Design review of the part built by this model. Coordinates are the model's own, in mm. A direction names the side the tool comes from. Give positions to 0.01 mm unless a question says otherwise; leave off trailing zeros. Write each loop counter-clockwise with the first axis right and the second up, starting at its lowest first coordinate (ties: lowest second). Pieces come first, ordered by that corner, then holes.
```python
from build123d import *

# Parameters (mm, degrees)
FILETE1_R = 2


with BuildPart() as part:
    # Esboço1 → Revolução1 (revolve)
    with BuildSketch(Plane.XY):
        Polygon((0, 31.5), (8, 31.5), (8, 27.5), (6, 27.5), (6, 0), (4, 0), (4, -21.5), (3.090074414, -24), (0, -24), align=None)
    revolve(axis=Axis((0, -53.197951274, 0), (0, 1, 0)))

    # Filete1
    filete1_edges = [part.edges().sort_by_distance(p)[0] for p in [
        (-8, 31.5, 0),
    ]]
    fillet(filete1_edges, radius=FILETE1_R)


solid = part.part
```
(1) Clearance check with flat-ended pins moving along their axes: P1, Ø4, axis at x = -6, y = 17.5, coming from the +Z side; P2, Ø5, axis at y = 16, z = -6, coming from the +X side; P3, Ø5, axis at y = 2, z = -2, coming from the +X side. State where each tip first meets the part, or that it passes through.
Resolved:
P1: stops at z = 4.47
P2: stops at x = 4.87
P3: stops at x = 6
(2) Consider section D-D, the plane y = 20. Give the boundary of the cut face in (x, z), then the cut area to 3 significant figures.
Resolved:
outline: circle Ø12 at (0, 0)
area: 113 mm2
(3) To check wall thickness, follow L1, parallel to Y at x = -0.5, z = -4.5; L2, parallel to X at y = -16.5, z = -2.75; L3, parallel to Z at x = -2.5, y = 12.5. State the ranges of each line that lie inside material, in increasing order.
Resolved:
L1: y = 0 to 31.5
L2: x = -2.9 to 2.9
L3: z = -5.45 to 5.45
(4) Consider section A-A, the plane z = 0. Give the boundary of the cut face in (x, y).
Resolved:
outline: (-8, 27.5) - (-6, 27.5) - (-6, 0) - (-4, 0) - (-4, -21.5) - (-3.09, -24) - (3.09, -24) - (4, -21.5) - (4, 0) - (6, 0) - (6, 27.5) - (8, 27.5) - (8, 29.5) arc R2 ccw to (6, 31.5) - (-6, 31.5) arc R2 ccw to (-8, 29.5) - close
(5) Tool access review of faces 1 (the face through (-6, 14, 0)), 2 (the face through (0, 31.5, 0)): name each direction out of +Z, -Z, +X, -X, +Y, -Y from which nothing blocks a thin tool from reaching the whole face with its end or side.
Resolved:
face 1: -Y
face 2: +Z, -Z, +X, -X, +Y
(6) Consider section C-C, the plane y = -15. Give the boundary of the cut face in (x, z), then the cut area to 3 significant figures.
Resolved:
outline: circle Ø8 at (0, 0)
area: 50.3 mm2
(7) Consider section B-B, the plane x = 0. Give the boundary of the cut face in (y, z), then the cut area to 3 significant figures.
Resolved:
outline: (-24, -3.09) - (-21.5, -4) - (0, -4) - (0, -6) - (27.5, -6) - (27.5, -8) - (29.5, -8) arc R2 ccw to (31.5, -6) - (31.5, 6) arc R2 ccw to (29.5, 8) - (27.5, 8) - (27.5, 6) - (0, 6) - (0, 4) - (-21.5, 4) - (-24, 3.09) - close
area: 582 mm2
